Read the model definition and answer for the solid it produces. Units are mm, in the model's axes. Face numbers are marked on the shaded views. A direction names the side the tool comes from. Give positions to 0.01 mm unless a question says otherwise; leave off trailing zeros. Order: outer loops, then holes, each group sorted by start corner. A loop starts at its lowest first (then second) coordinate and runs counter-clockwise, first axis right, second up. Notation, with made-up numbers: (78.5, 30) - (120.5, 30) arc R15 ccw to (120.5, 53) - close; hole circle Ø8 at (-30, 54.5). An arc over 180 degrees is marked (long way). Use a Markdown table: item, result. Add a question column.
1. A cutting plane is placed at D-D on z = 0.9. State how many separate pieces and enclosed holes the cut face has, and give its area (3 significant figures).
2. For a pull along X with two mould halves and no side action, classify the marked faces 1, 2 and 3 as released by +X, released by -X, zero draft, split by the parting line, or undercut.
3. Consider L1, parallel to Y at x = 3.4, z = 0.6; L2, parallel to X at y = 3.4, z = 1.05; L3, parallel to X at y = 34, z = 1.15. Determine where each line is inside the solid, lowest interval first.
4. Flat-ended cylindrical pins translate along their axes: P1, Ø1, axis at y = 4, z = 2.5, coming from the -X side; P2, Ø1, axis at x = -14, z = 1.5, coming from the +Y side; P3, Ø1, axis at x = -6.5, z = 2, coming from the +Y side; P4, Ø4, axis at x = -9.29, y = 34.19, coming from the +Z side. Find the tip coordinate at first contact, or state that the pin passes through.
5. A cutting plane is placed at A-A on x = 7.5. Determine the outline of the cut face in (y, z).
6. A cutting plane is placed at C-C on x = 3.4. Determine the outline of the cut face in (y, z).
7. A cutting plane is placed at B-B on y = 7.5. Determine the outline of the cut face in (x, z), and give its area (3 significant figures).
8. Which of the six approach directions +Z, -Z, +X, -X, +Y, -Y give full straight-line access (tool end or side, diameter ignored) to the marked faces 4 and 5?
```python
from build123d import *

# Parameters (mm, degrees)
BOSS_EXTRUDE1_OUTLINE_R   = 1.5
BOSS_EXTRUDE1_OUTLINE_R_2 = 2.625
BOSS_EXTRUDE1_DEPTH       = 3.05


# Read off the part's stored shape, not the designer's step: Boss-Extrude1
with BuildPart() as part:
    # Boss-Extrude1 outline → Boss-Extrude1 (new body)
    with BuildSketch(Plane.XY):
        with BuildLine():
            ThreePointArc((-5.096612315, 30.628825091), (-6.864545193, 39.127004069), (-14.669149283, 35.327953187))
            add(Edge.make_bspline(
                [(-18.236074249, 29.557782775), (-15.56964568, 31.860427367), (-14.669149283, 35.327953187)],
                knots=[0, 0, 0, 1, 1, 1], degree=2))
            Line((-18.236074249, 29.557782775), (-20.68803125, 27.733458745))
            Line((-20.68803125, 27.733458745), (-18.748011912, 25.126003095))
            Line((-18.748011912, 25.126003095), (-14.872658256, 28.009373723))
            add(Edge.make_bspline(
                [(-14.872658256, 28.009373723), (-13.321413482, 29.087354752), (-12.034218378, 29.87005609), (-10.324464656, 28.408317489), (-8.803360363, 24.654236343)],
                knots=[0, 0, 0, 0, 0.517103648, 1, 1, 1, 1], degree=3))
            Line((-8.803360363, 24.654236343), (0, 0))
            Line((0, 0), (13, 0))
            Line((13, 0), (13, 6.303908615))
            Line((13, 6.303908615), (-0.225000063, 16.985639436))
            Line((-0.225000063, 16.985639436), (-5.096612315, 30.628825091))
        make_face()
        with Locations((3.4, 3.4)):
            Circle(BOSS_EXTRUDE1_OUTLINE_R, mode=Mode.SUBTRACT)
        Polygon((3.95568576, 11.322036253), (11.073847559, 5.572751724), (9.063168816, 3.083339947), (1.945007017, 8.832624477), align=None, mode=Mode.SUBTRACT)
        with Locations((-9.28819898, 34.189808273)):
            Circle(BOSS_EXTRUDE1_OUTLINE_R_2, mode=Mode.SUBTRACT)
    extrude(amount=BOSS_EXTRUDE1_DEPTH)

    # Sketch3 → CSK for M3 Flat Head Machine Screw1 (revolve, cut)
    with BuildSketch(Plane(origin=(3.4, 3.4, 3.05), x_dir=(0, -1, 0), z_dir=(1, 0, 0))):
        Polygon((0, 0), (0, 3.05), (1.55, 3.05), (1.55, 1.6), (3.15, 0), align=None)
    revolve(axis=Axis((3.4, 3.4, 9.4), (0, 0, -1)), mode=Mode.SUBTRACT)


solid = part.part
```
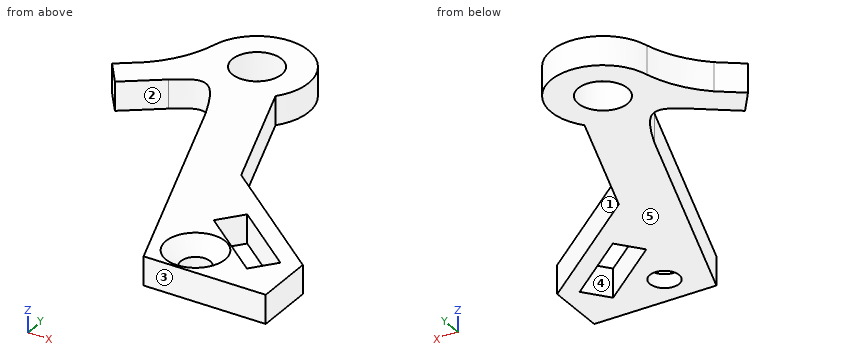
Output values:
| question | item | result |
|---|---|---|
| 1 | separate pieces | 1 |
| 1 | enclosed holes | 3 |
| 1 | area | 339 mm² |
| 2 | face 1 | released by +X |
| 2 | face 2 | undercut |
| 2 | face 3 | zero draft |
| 3 | L1 | 0 to 1.85, 4.95 to 7.66, 10.63 to 14.06 |
| 3 | L2 | -1.21 to 1.85, 4.95 to 8.67, 9.32 to 13 |
| 3 | L3 | -15.1 to -11.91, -6.67 to -3.79 |
| 4 | P1 | x = -1.61 |
| 4 | P2 | y = 37.73 |
| 4 | P3 | y = 39.19 |
| 4 | P4 | through |
| 5 | outline | (0, 0) - (4.35, 0) - (4.35, 3.05) - (0, 3.05) - close; (8.46, 0) - (10.75, 0) - (10.75, 3.05) - (8.46, 3.05) - close |
| 6 | outline | (0, 0) - (1.85, 0) - (1.85, 1.45) - (0.25, 3.05) - (0, 3.05) - close; (4.95, 0) - (7.66, 0) - (7.66, 3.05) - (6.55, 3.05) - (4.95, 1.45) - close; (10.63, 0) - (14.06, 0) - (14.06, 3.05) - (10.63, 3.05) - close |
| 7 | outline | (-2.68, 0) - (3.59, 0) - (3.59, 3.05) - (-2.68, 3.05) - close; (8.69, 0) - (11.52, 0) - (11.52, 3.05) - (8.69, 3.05) - close |
| 7 | area | 27.8 mm² |
| 8 | face 4 | +Z, -Z |
| 8 | face 5 | -Z, +X, -X, +Y, -Y |
